Drawing for the job (mm, zero at the part's lowest x, y, z). Coordinates: 2 decimals unless noted, no trailing zeros. Order: outer loops, then holes, each group sorted by start corner. A loop starts at its lowest first (then second) coordinate and runs counter-clockwise, first axis right, second up.
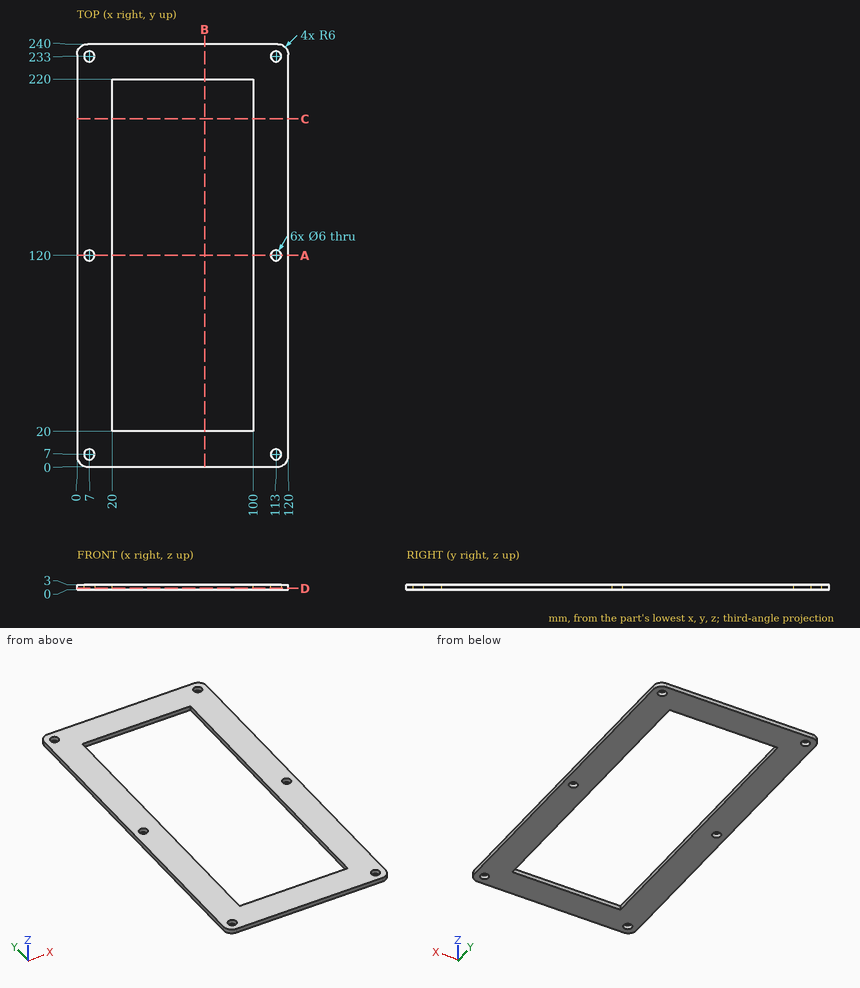
(1) Slice it at B-B, the plane x = 72.5. Give the cut face in (y, z).
(2) Slice it at D-D, the plane z = 0.85. Give the cut face in (x, y).
(3) Probe line 1 (Y direction, x = 7, z = 1.4); line 2 (Y direction, x = 68.5, z = 1.75); line 3 (X direction, y = 95.5, z = 2.2). List the from-to ranges inside material, lowest first.
(4) Slice it at C-C, the plane y = 197.5. Give the cut face in (x, z), then the cut area to 3 significant figures.
(5) Slice it at A-A, the plane y = 120. Give the cut face in (x, z), then the cut area to 3 significant figures.
Here are the results:
1. outline: (0, 0) - (20, 0) - (20, 3) - (0, 3) - close; (220, 0) - (240, 0) - (240, 3) - (220, 3) - close
2. outline: (0, 6) arc R6 ccw to (6, 0) - (114, 0) arc R6 ccw to (120, 6) - (120, 234) arc R6 ccw to (114, 240) - (6, 240) arc R6 ccw to (0, 234) - close; hole circle Ø6 at (7, 7); hole circle Ø6 at (7, 120); hole circle Ø6 at (7, 233); hole (20, 20) - (100, 20) - (100, 220) - (20, 220) - close; hole circle Ø6 at (113, 7); hole circle Ø6 at (113, 120); hole circle Ø6 at (113, 233)
3. line 1: y = 0 to 4, 10 to 117, 123 to 230, 236 to 240
3. line 2: y = 0 to 20, 220 to 240
3. line 3: x = 0 to 20, 100 to 120
4. outline: (0, 0) - (20, 0) - (20, 3) - (0, 3) - close; (100, 0) - (120, 0) - (120, 3) - (100, 3) - close
4. area: 120 mm2
5. outline: (0, 0) - (4, 0) - (4, 3) - (0, 3) - close; (10, 0) - (20, 0) - (20, 3) - (10, 3) - close; (100, 0) - (110, 0) - (110, 3) - (100, 3) - close; (116, 0) - (120, 0) - (120, 3) - (116, 3) - close
5. area: 84.0 mm2
